For this review, use the dimensioned drawing (mm, ordinates from the lowest corner) and the shaded views. A direction names the side the tool comes from. Coordinates: 2 decimals unless noted, no trailing zeros. Loops run counter-clockwise (first coordinate to the right, second up) from the corner with the lowest first, then second, coordinate; pieces in that order, holes last. Notation, with made-up numbers: (-29.5, 50.25) -> (26.5, 50.25) arc R9 ccw to (26.5, 59.25) -> close; hole circle Ø5 at (10, 14.25). An arc over 180 degrees is marked (long way). Use one line per item in the form item = value. Start each with the question number.
1. Consider section A-A (y = 9.5). State the section outline as (x, z) points.
2. For pin 1 (7.5 mm diameter, centred on x = 12.5, z = 20.5, fed in from -Y); pin 2 (3 mm diameter, centred on x = 24, z = 34, fed in from -Y); pin 3 (2.5 mm diameter, centred on x = 3.5, z = 31.05, fed in from +Y), all flat-tipped, find the tip position at first contact; note any pin that passes through.
3. The part is to be moulded in two halves that separate along X. For the marked faces 3, 4 and 5, say which applies: released by +X, released by -X, zero draft, split by the parting line, or undercut.
4. Consider section D-D (z = 21). State the section outline as (x, y) points.
5. Wall thickness on line 1 (X direction, y = 1, z = 8); line 2 (Z direction, x = 3.5, y = 7.4); line 3 (Y direction, x = 13, z = 16): over which ranges is each line inside the solid? List them lowest first. Write a range as from..to.
6. Consider section C-C (x = 28.5). State the section outline as (y, z) points.
7. Consider section B-B (y = 4). State the section outline as (x, z) points.
8. Machinability: for the marked faces 1 and 2, which of the approach directions +Z, -Z, +X, -X, +Y, -Y give a long, thin tool a straight path to every point of the face, cutting with its end or side? Answer none if there is none.
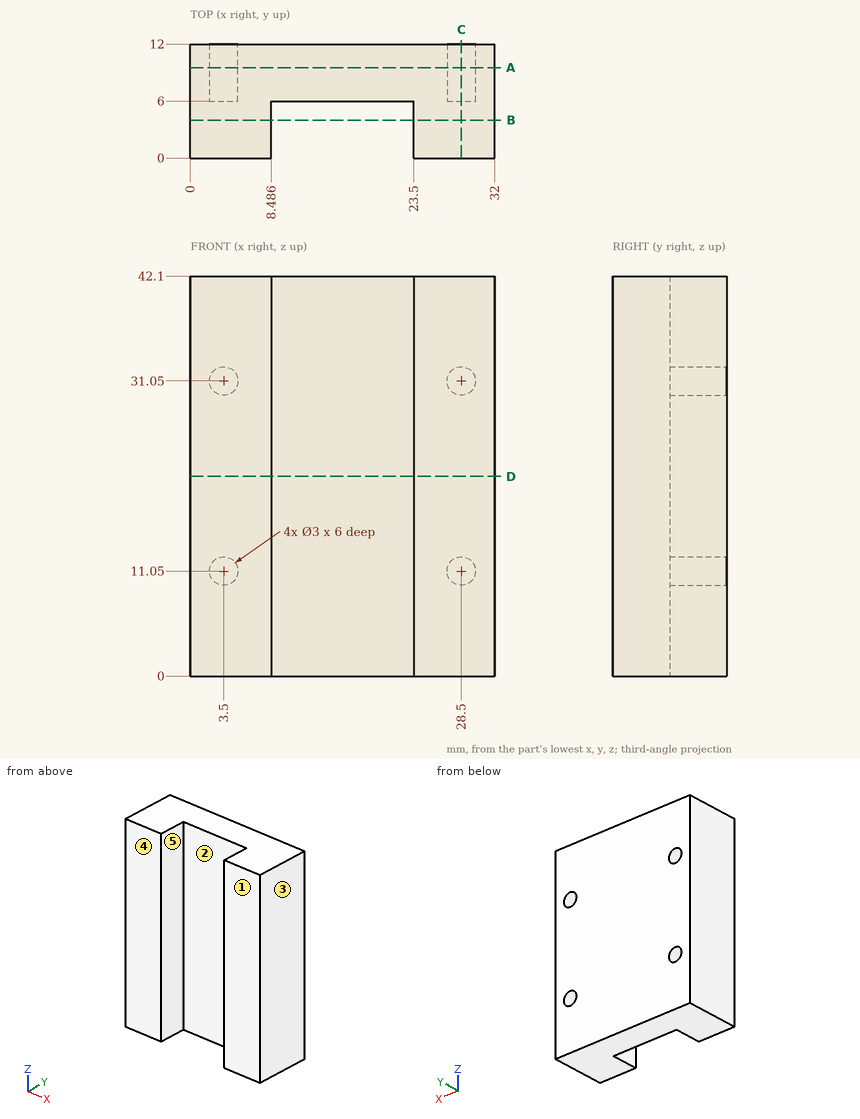
Geometry check:
q1.outline = (0, 0) -> (32, 0) -> (32, 42.1) -> (0, 42.1) -> close; hole circle Ø3 at (3.5, 11.05); hole circle Ø3 at (3.5, 31.05); hole circle Ø3 at (28.5, 11.05); hole circle Ø3 at (28.5, 31.05)
q2.pin_1 = 6
q2.pin_2 = 0
q2.pin_3 = 6
q3.face_3 = released by +X
q3.face_4 = zero draft
q3.face_5 = undercut
q4.outline = (0, 0) -> (8.49, 0) -> (8.49, 6) -> (23.5, 6) -> (23.5, 0) -> (32, 0) -> (32, 12) -> (0, 12) -> close
q5.line_1 = 0..8.49, 23.5..32
q5.line_2 = 0..9.55, 12.55..29.55, 32.55..42.1
q5.line_3 = 6..12
q6.outline = (0, 0) -> (12, 0) -> (12, 9.55) -> (6, 9.55) -> (6, 12.55) -> (12, 12.55) -> (12, 29.55) -> (6, 29.55) -> (6, 32.55) -> (12, 32.55) -> (12, 42.1) -> (0, 42.1) -> close
q7.outline = (0, 0) -> (8.49, 0) -> (8.49, 42.1) -> (0, 42.1) -> close; (23.5, 0) -> (32, 0) -> (32, 42.1) -> (23.5, 42.1) -> close
q8.face_1 = +Z, -Z, +X, -X, -Y
q8.face_2 = +Z, -Z, -Y
